Part model, mm, in its own coordinate system. A direction names the side the tool comes from. Round coordinates to 2 decimals unless told otherwise and drop trailing zeros. Write each loop counter-clockwise with the first axis right and the second up, starting at its lowest first coordinate (ties: lowest second). Pieces come first, ordered by that corner, then holes. Notation, with made-up numbers: (-35.75, -12.5) -> (-14.75, -12.5) arc R19 cw to (-14.75, -3.5) -> close; hole circle Ø8 at (-18.75, 47). An arc over 180 degrees is marked (long way). Return JSON: item names as keys, results as strings. Group by question number.
```python
from build123d import *

# Parameters (mm, degrees)
BOSS_EXTRUDE1_DEPTH = 2
SKETCH2_W           = 110.931662833
SKETCH2_H           = 3
SKETCH2_W_2         = 124.512387616
SKETCH2_W_3         = 131.50444394
SKETCH2_W_4         = 133.924771129
CUT_EXTRUDE1_DEPTH  = 0.5


with BuildPart() as part:
    # Sketch1 → Boss-Extrude1 (new body)
    with BuildSketch(Plane(origin=(0, 0, 0), x_dir=(1, 0, 0), z_dir=(0, 1, 0))):
        with BuildLine():
            Line((0, 35), (-60, 35))
            ThreePointArc((-60, 35), (-95, 0), (-60, -35))
            Line((-60, -35), (0, -35))
            ThreePointArc((0, -35), (35, 0), (0, 35))
        make_face()
    extrude(amount=BOSS_EXTRUDE1_DEPTH)

    # Sketch2 → Cut-Extrude1 (cut)
    with BuildSketch(Plane(origin=(0, 2, 0), x_dir=(1, 0, 0), z_dir=(0, 1, 0))):
        with Locations((-30.336156555, 28.5)):
            Rectangle(SKETCH2_W, SKETCH2_H)
        with Locations((-30, 20.5)):
            Rectangle(SKETCH2_W_2, SKETCH2_H)
        with Locations((-29.865537378, 12.5)):
            Rectangle(SKETCH2_W_3, SKETCH2_H)
        with Locations((-28.655373784, 4.5)):
            Rectangle(SKETCH2_W_4, SKETCH2_H)
        with Locations((-28.655373784, -4.5)):
            Rectangle(SKETCH2_W_4, SKETCH2_H)
        with Locations((-29.865537378, -12.5)):
            Rectangle(SKETCH2_W_3, SKETCH2_H)
        with Locations((-30, -20.5)):
            Rectangle(SKETCH2_W_2, SKETCH2_H)
        with Locations((-30.336156555, -28.5)):
            Rectangle(SKETCH2_W, SKETCH2_H)
    extrude(amount=-CUT_EXTRUDE1_DEPTH, mode=Mode.SUBTRACT)


solid = part.part
```
Item 1: Wall check: L1, parallel to X at y = 0.4, z = -11; L2, parallel to Y at x = 29, z = 11.5; L3, parallel to Z at x = 18, y = 0.65. Give the ranges that are in metal, low to high.
Item 2: Flat gauge pins, fed straight in: P1, Ø0.6, axis at x = -60.5, y = 2, coming from the +Z side; P2, Ø1, axis at x = -70, z = 12, coming from the +Y side. Where does each tip first touch, or does it go through?
Item 3: Cut at A-A (y = 1.05). Write the cut outline in (x, z).
Item 4: Cut at B-B (x = 25). Write the cut outline in (y, z).
Item 5: Which spindle directions (+Z, -Z, +X, -X, +Y, -Y) get a long thin tool onto all of the face, cutting with end or side? Do faces 4 (the face through (-31, 2, -17)), 5 (the face through (-31, 1.5, -29)). Say none if no direction does.
Item 6: Cut at C-C (z = -8.5). Write the cut outline in (x, y), then the cut area to 3 significant figures.
Item 7: Two-plate mould, pull along Z, no slides. Class faces 1 (the face through (-31, 2, -33)), 2 (the face through (-94.99, 0.99, -0.77)), 3 (the face through (-31, 1.5, 4)): released by +Z, released by -Z, zero draft, split by the parting line, or undercut.
Checks:
{
 "1": {"L1": "x = -93.23 to 33.23", "L2": "y = 0 to 1.5", "L3": "z = -30.02 to 30.02"},
 "2": {"P1": "stops at z = 35", "P2": "stops at y = 1.5"},
 "3": {"outline": "(-60, -35) -> (0, -35) arc R35 ccw to (0, 35) -> (-60, 35) arc R35 ccw to start"},
 "4": {"outline": "(0, -24.49) -> (2, -24.49) -> (2, -22) -> (1.5, -22) -> (1.5, -19) -> (2, -19) -> (2, -14) -> (1.5, -14) -> (1.5, -11) -> (2, -11) -> (2, -6) -> (1.5, -6) -> (1.5, -3) -> (2, -3) -> (2, 3) -> (1.5, 3) -> (1.5, 6) -> (2, 6) -> (2, 11) -> (1.5, 11) -> (1.5, 14) -> (2, 14) -> (2, 19) -> (1.5, 19) -> (1.5, 22) -> (2, 22) -> (2, 24.49) -> (0, 24.49) -> close"},
 "5": {"face 4": "+Z, -Z, +X, -X, +Y", "face 5": "+X, -X, +Y"},
 "6": {"outline": "(-93.95, 0) -> (33.95, 0) -> (33.95, 2) -> (-93.95, 2) -> close", "area": "256 mm2"},
 "7": {"face 1": "zero draft", "face 2": "split by the parting line", "face 3": "undercut"}
}
